Autodesk Fusion 360 part; units mm, degrees
sketch "Switch" plane through (0, 0, 0) normal (0, 1, 0) x (1, 0, 0)
  line L0 (-7.1721, 7.2) -> (7.2279, 7.2)
  line L1 (-8.6721, -8.7) -> (-8.6721, 8.7)
  line L2 (7.2279, -7.2) -> (-7.1721, -7.2)
  line L3 (-8.6721, 8.7) -> (8.7279, 8.7)
  line L4 (-8.6721, -8.7) -> (8.7279, 8.7) construction
  line L5 (-7.1721, -7.2) -> (7.2279, 7.2) construction
  line L6 (8.7279, -8.7) -> (-8.6721, -8.7)
  line L7 (-7.1721, -7.2) -> (-7.1721, 7.2)
  line L8 (7.2279, 7.2) -> (7.2279, -7.2)
  line L9 (8.7279, 8.7) -> (8.7279, -8.7)
  line L10 (8.7279, -8.7) -> (-8.6721, 8.7) construction
  line L11 (7.2279, -7.2) -> (-7.1721, 7.2) construction
  line L12 (-12, 12) -> (12, 12)
  line L13 (12, 12) -> (12, -12)
  line L14 (12, -12) -> (-12, -12)
  line L15 (-12, -12) -> (-12, 12)
  line L16 (-12, 12) -> (12, -12) construction
  line L17 (12, 12) -> (-12, -12) construction
  point P0 (0.0279, 0)
  dimension "d1" = 14.4
  dimension "d2" = 14.4
  dimension "d3" = 1.5
  dimension "d4" = 1.5
  dimension "d5" = 1.5
  dimension "d6" = 1.5
  dimension "d7" = 24
  dimension "d8" = 24
extrude "Extrude1" add sketch "Switch" along normal blind 3 contours L12 L13 L14 L15
extrude "Extrude2" add sketch "Switch" along normal blind 1.3 contours L1 L3 L6 L9
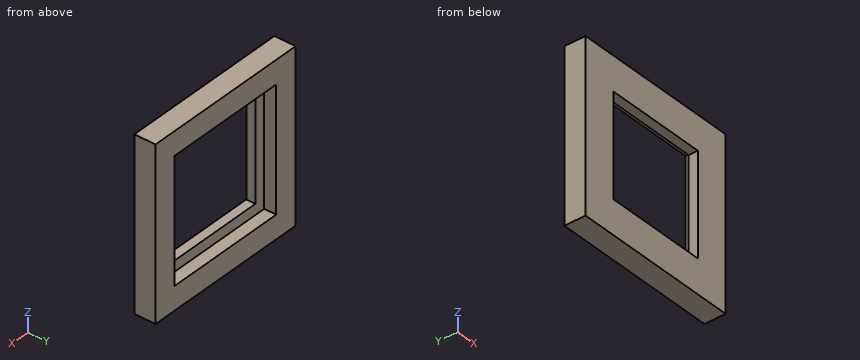
Source: CAD feature listing. Evaluate the final solid. Frame: model axes, mm. Round coordinates to 2 decimals unless told otherwise and drop trailing zeros. Loops run counter-clockwise (first coordinate to the right, second up) from the corner with the lowest first, then second, coordinate; pieces in that order, holes last. Notation, with made-up numbers: M -13,67.5 L -3,67.5 A15 cw -3,93.5 Z; hole C 21,80 d6. An arc over 180 degrees is marked long. Use a Markdown table: item, result. Add a question column.
1. Contact query for flat-ended pins moving along their axis: pin 1 (6 mm diameter, centred on x = -8, z = -8.5, fed in from -Y); pin 2 (8.5 mm diameter, centred on x = -3.5, z = 0, fed in from +Y). Output: stop coordinate, or through.
2. Cut plane C-C, the plane z = 8.25. Output: boundary loops of the cut face in (x, y), and give its area (3 significant figures).
3. Cut plane D-D, the plane y = 0.5. Output: boundary loops of the cut face in (x, z), and give its area (3 significant figures).
4. Cut plane B-B, the plane y = 2.4. Output: boundary loops of the cut face in (x, z), and give its area (3 significant figures).
5. Ray query, line 1 along X through (y, z) = (1.6, -1.75); line 2 along Z through (x, y) = (7.75, 2.7); line 3 along Z through (x, y) = (-4.5, 1.05). Return the intervals inside material, ascending. Write a range as [from, to].
6. Cut plane A-A, the plane x = 0.75. Output: boundary loops of the cut face in (y, z), and give its area (3 significant figures).
Solution:
| question | item | result |
|---|---|---|
| 1 | pin 1 | stops at y = 0 |
| 1 | pin 2 | stops at y = 1.3 |
| 2 | outline | M -12,0 L 12,0 L 12,3 L 8.73,3 L 8.73,1.3 L -8.67,1.3 L -8.67,3 L -12,3 Z |
| 2 | area | 42.4 mm2 |
| 3 | outline | M -12,-12 L 12,-12 L 12,12 L -12,12 Z; hole M -7.17,-7.2 L 7.23,-7.2 L 7.23,7.2 L -7.17,7.2 Z |
| 3 | area | 369 mm2 |
| 4 | outline | M -12,-12 L 12,-12 L 12,12 L -12,12 Z; hole M -8.67,-8.7 L 8.73,-8.7 L 8.73,8.7 L -8.67,8.7 Z |
| 4 | area | 273 mm2 |
| 5 | line 1 | x = [-12, -8.67], [8.73, 12] |
| 5 | line 2 | z = [-12, -8.7], [8.7, 12] |
| 5 | line 3 | z = [-12, -7.2], [7.2, 12] |
| 6 | outline | M 0,-12 L 3,-12 L 3,-8.7 L 1.3,-8.7 L 1.3,-7.2 L 0,-7.2 Z; M 0,7.2 L 1.3,7.2 L 1.3,8.7 L 3,8.7 L 3,12 L 0,12 Z |
| 6 | area | 23.7 mm2 |
